Here's how the part is built. I have some questions about the finished solid (model axes, mm). A direction names the side the tool comes from. Coordinates: 2 decimals unless noted, no trailing zeros. Order: outer loops, then holes, each group sorted by start corner. A loop starts at its lowest first (then second) coordinate and runs counter-clockwise, first axis right, second up. Notation, with made-up numbers: (57.5, -10.5) -> (66.5, -10.5) arc R22 cw to (66.5, 7.5) -> close; hole circle Ø11 at (-38.5, 67). An arc over 180 degrees is marked (long way). One line per item, written item: value. Start each with the question number.
```python
from build123d import *

# Parameters (mm, degrees)
F0_R     = 3.1
F1_DEPTH = 10


with BuildPart() as f1:
    # F0 (on Top) → F1 (new body)
    with BuildSketch(Plane.XY):
        with BuildLine():
            ThreePointArc((1.673929859, 12.3874113045), (0, 12.5), (-1.673929859, 12.3874113045))
            ThreePointArc((-1.673929859, 12.3874113045), (-3.7588224938, 11.9214618844), (-5.7339241657, 11.1073000167))
            ThreePointArc((-5.7339241657, 11.1073000167), (-7.1697054544, 10.2394005536), (-8.4763302976, 9.1870465703))
            ThreePointArc((-8.4763302976, 9.1870465703), (-9.9902333855, 7.5130045191), (-11.1784184623, 5.5940111443))
            ThreePointArc((-11.1784184623, 5.5940111443), (-11.8268519609, 4.0466742757), (-12.2622342862, 2.4264398427))
            ThreePointArc((-12.2622342862, 2.4264398427), (-12.4986778991, 0.1817987206), (-12.3276190694, -2.0687697022))
            ThreePointArc((-12.3276190694, -2.0687697022), (-11.9395449954, -3.7009816676), (-11.336389674, -5.2665234414))
            ThreePointArc((-11.336389674, -5.2665234414), (-10.2045206414, -7.2192630149), (-8.7399470524, -8.9366283084))
            ThreePointArc((-8.7399470524, -8.9366283084), (-7.4644823963, -10.0265399094), (-6.0545511265, -10.9358315027))
            ThreePointArc((-6.0545511265, -10.9358315027), (-3.9892887467, -11.8463317232), (-1.7939610174, -12.3705983634))
            ThreePointArc((-1.7939610174, -12.3705983634), (-0.1212015211, -12.4994123938), (1.5537413227, -12.4030596186))
            ThreePointArc((1.5537413227, -12.4030596186), (3.7588224938, -11.9214618844), (5.8413523551, -11.0511810529))
            ThreePointArc((5.8413523551, -11.0511810529), (7.2686508911, -10.1694008783), (8.5650105596, -9.1044271711))
            ThreePointArc((8.5650105596, -9.1044271711), (10.0626107657, -7.4157848255), (11.2321331944, -5.4853608726))
            ThreePointArc((11.2321331944, -5.4853608726), (11.8655330447, -3.9318094519), (12.285184913, -2.3074296637))
            ThreePointArc((12.285184913, -2.3074296637), (12.4998530976, -0.0606014727), (12.3069805238, 2.188202547))
            ThreePointArc((12.3069805238, 2.188202547), (11.9030985667, 3.8165749712), (11.2847919153, 5.3761948838))
            ThreePointArc((11.2847919153, 5.3761948838), (10.1340420896, 7.3178679221), (8.6528855651, 9.0209518011))
            ThreePointArc((8.6528855651, 9.0209518011), (7.3669129512, 10.0984451065), (5.9482313582, 10.9940230903))
            ThreePointArc((5.9482313582, 10.9940230903), (3.8742377423, 11.8844554741), (1.673929859, 12.3874113045))
        make_face()
        Circle(F0_R, mode=Mode.SUBTRACT)
        with BuildLine():
            ThreePointArc((-12.2622342862, 2.4264398427), (-11.8268519609, 4.0466742757), (-11.1784184623, 5.5940111443))
            Line((-11.1784184623, 5.5940111443), (-14.1805287895, 6.6212128607))
            ThreePointArc((-14.1805287895, 6.6212128607), (-15.0512360756, 6.1003265438), (-15.786995451, 5.4016765064))
            ThreePointArc((-15.786995451, 5.4016765064), (-15.6334500279, 4.3987420438), (-15.2643446134, 3.4536415591))
            Line((-15.2643446134, 3.4536415591), (-12.2622342862, 2.4264398427))
        make_face()
        with BuildLine():
            ThreePointArc((-11.336389674, -5.2665234414), (-11.9395449954, -3.7009816676), (-12.3276190694, -2.0687697022))
            Line((-12.3276190694, -2.0687697022), (-15.3583352271, -3.0082213265))
            ThreePointArc((-15.3583352271, -3.0082213265), (-15.7547724734, -3.9421866593), (-15.9374230058, -4.9402310051))
            ThreePointArc((-15.9374230058, -4.9402310051), (-15.2222949332, -5.6599848332), (-14.3671058317, -6.2059750657))
            Line((-14.3671058317, -6.2059750657), (-11.336389674, -5.2665234414))
        make_face()
        with BuildLine():
            ThreePointArc((-6.0545511265, -10.9358315027), (-7.4644823963, -10.0265399094), (-8.7399470524, -8.9366283084))
            Line((-8.7399470524, -8.9366283084), (-10.6347200455, -11.4817501301))
            ThreePointArc((-10.6347200455, -11.4817501301), (-10.4045567225, -12.4699194364), (-9.9639151672, -13.3838607655))
            ThreePointArc((-9.9639151672, -13.3838607655), (-8.9619915366, -13.5438694265), (-7.9493241196, -13.4809533245))
            Line((-7.9493241196, -13.4809533245), (-6.0545511265, -10.9358315027))
        make_face()
        with BuildLine():
            ThreePointArc((1.5537413227, -12.4030596186), (-0.1212015211, -12.4994123938), (-1.7939610174, -12.3705983634))
            Line((-1.7939610174, -12.3705983634), (-1.8247266294, -15.5434304201))
            ThreePointArc((-1.8247266294, -15.5434304201), (-1.0564027139, -16.2061008466), (-0.1617850522, -16.6847583155))
            ThreePointArc((-0.1617850522, -16.6847583155), (0.7419462008, -16.2235386762), (1.5229757107, -15.5758916753))
            Line((1.5229757107, -15.5758916753), (1.5537413227, -12.4030596186))
        make_face()
        with BuildLine():
            Line((10.4100739777, -11.6858126065), (8.5650105596, -9.1044271711))
            ThreePointArc((8.5650105596, -9.1044271711), (7.2686508911, -10.1694008783), (5.8413523551, -11.0511810529))
            Line((5.8413523551, -11.0511810529), (7.6864157733, -13.6325664882))
            ThreePointArc((7.6864157733, -13.6325664882), (8.6976727518, -13.71510773), (9.7025107722, -13.5745577889))
            ThreePointArc((9.7025107722, -13.5745577889), (10.1607920135, -12.6693329344), (10.4100739777, -11.6858126065))
        make_face()
        with BuildLine():
            Line((15.2971139884, -3.3054742658), (12.285184913, -2.3074296637))
            ThreePointArc((12.285184913, -2.3074296637), (11.8655330447, -3.9318094519), (11.2321331944, -5.4853608726))
            Line((11.2321331944, -5.4853608726), (14.2440622698, -6.4834054748))
            ThreePointArc((14.2440622698, -6.4834054748), (15.1096780482, -5.9541011602), (15.8386286408, -5.2483499528))
            ThreePointArc((15.8386286408, -5.2483499528), (15.6753658611, -4.2469514318), (15.2971139884, -3.3054742658))
        make_face()
        with BuildLine():
            Line((14.3062565663, 6.3449885386), (11.2847919153, 5.3761948838))
            ThreePointArc((11.2847919153, 5.3761948838), (11.9030985667, 3.8165749712), (12.3069805238, 2.188202547))
            Line((12.3069805238, 2.188202547), (15.3284451748, 3.1569962018))
            ThreePointArc((15.3284451748, 3.1569962018), (15.7158079437, 4.0947615341), (15.8887727305, 5.0945299651))
            ThreePointArc((15.8887727305, 5.0945299651), (15.1666994543, 5.8073159898), (14.3062565663, 6.3449885386))
        make_face()
        with BuildLine():
            Line((7.81823747, 13.5573972192), (5.9482313582, 10.9940230903))
            ThreePointArc((5.9482313582, 10.9940230903), (7.3669129512, 10.0984451065), (8.6528855651, 9.0209518011))
            Line((8.6528855651, 9.0209518011), (10.5228916769, 11.58432593))
            ThreePointArc((10.5228916769, 11.58432593), (10.2831577637, 12.5702170924), (9.833675236, 13.4798429443))
            ThreePointArc((9.833675236, 13.4798429443), (8.8302472408, 13.6301293101), (7.81823747, 13.5573972192))
        make_face()
        with BuildLine():
            Line((-1.673929859, 15.5603925183), (-1.673929859, 12.3874113045))
            ThreePointArc((-1.673929859, 12.3874113045), (0, 12.5), (1.673929859, 12.3874113045))
            Line((1.673929859, 12.3874113045), (1.673929859, 15.5603925183))
            ThreePointArc((1.673929859, 15.5603925183), (0.8992167282, 16.2155820315), (0, 16.6855426777))
            ThreePointArc((0, 16.6855426777), (-0.8992167282, 16.2155820315), (-1.673929859, 15.5603925183))
        make_face()
        with BuildLine():
            ThreePointArc((-8.4763302976, 9.1870465703), (-7.1697054544, 10.2394005536), (-5.7339241657, 11.1073000167))
            Line((-5.7339241657, 11.1073000167), (-7.5538714229, 13.7064540645))
            ThreePointArc((-7.5538714229, 13.7064540645), (-8.5642805338, 13.7987966969), (-9.5704341076, 13.6679963945))
            ThreePointArc((-9.5704341076, 13.6679963945), (-10.0374709761, 12.767257644), (-10.2962775548, 11.7862006181))
            Line((-10.2962775548, 11.7862006181), (-8.4763302976, 9.1870465703))
        make_face()
    extrude(amount=F1_DEPTH)


solid = f1.part
```
Q1. Imagine slicing it at C-C (y = 10). Write out the boundary of the cut face in (x, z).
Q2. For faces 1 (the face through (-12.87, -5.74, 4.93)), 2 (the face through (-10, 7.5, 4.9)), 3 (the face through (-13.784, 2.947, 4.93)), 4 (the face through (15.68, -4.26, 4.93)), which set-ups out of +Z, -Z, +X, -X, +Y, -Y let a thin tool reach every point of the face, with its end or its side?
Q3. I need wall thicknesses on line 1 (X direction, y = -11, z = 4.75); line 2 (Y direction, x = -7.5, z = 7.75); line 3 (Y direction, x = -6, z = 6.25). Which ranges of each line are inside material? Lowest first, please.
Q4. If we mould it in two halves opening along Y, with no side actions, what happens to faces 5 (the face through (3.73, -11.93, 4.93)), 6 (the face through (10.288, 12.557, 4.93)), 7 (the face through (-9.399, 10.505, 4.93))? For each: +Y half, -Y half, draft (parallel to the pull), parting line (faces both ways), or undercut.
Q5. For P1, Ø1.6, axis at y = 14.5, z = 5, coming from the +X side; P2, Ø5, axis at x = 7.5, z = 4.5, coming from the +Y side; P3, Ø2, axis at y = -10, z = 2, coming from the -X side, each with a flat end and sliding along its axis, tell me the tip position at first contact or that it passes through.
Q6. Imagine slicing it at A-A (y = 0). Write out the boundary of the cut face in (x, z), plus the area to 3 significant figures.
Q7. Imagine slicing it at B-B (x = 1). Write out the boundary of the cut face in (y, z), plus the area to 3 significant figures.
Completed:
1. outline: (-9.05, 0) -> (9.37, 0) -> (9.37, 10) -> (-9.05, 10) -> close
2. face 1: +Z, -Z, -Y
2. face 2: +Z, -Z
2. face 3: +Z, -Z, -X
2. face 4: +Z, -Z, +X
3. line 1: x = -10.28 to -6.1, -5.94 to 9.92
3. line 2: y = -12.88 to 13.63
3. line 3: y = -10.97 to 11.49
4. face 5: -Y half
4. face 6: +Y half
4. face 7: undercut
5. P1: stops at x = 1.67
5. P2: stops at y = 13.63
5. P3: stops at x = -10.28
6. outline: (-12.5, 0) -> (-3.1, 0) -> (-3.1, 10) -> (-12.5, 10) -> close; (3.1, 0) -> (12.5, 0) -> (12.5, 10) -> (3.1, 10) -> close
6. area: 188 mm2
7. outline: (-16.04, 0) -> (-2.93, 0) -> (-2.93, 10) -> (-16.04, 10) -> close; (2.93, 0) -> (16.15, 0) -> (16.15, 10) -> (2.93, 10) -> close
7. area: 263 mm2
